from build123d import *

# Parameters (mm, degrees)
SKETCH1_R           = 38.1
BOSS_EXTRUDE1_DEPTH = 12.7
SKETCH2_R           = 24.13
CUT_EXTRUDE1_DEPTH  = 5.08


with BuildPart() as part:
    # Sketch1 → Boss-Extrude1 (new body)
    with BuildSketch(Plane(origin=(0, 0, 0), x_dir=(1, 0, 0), z_dir=(0, 1, 0))):
        with Locations(Location((0, 0, 0), (0, 0, 270))):
            Circle(SKETCH1_R)
    boss_extrude1 = extrude(amount=BOSS_EXTRUDE1_DEPTH)

    # Sketch2 → Cut-Extrude1 (cut)
    with BuildSketch(Plane(origin=(0, 12.7, 0), x_dir=(1, 0, 0), z_dir=(0, 1, 0))):
        with Locations(Location((0, 0, 0), (0, 0, 270))):
            Circle(SKETCH2_R)
    cut_extrude1 = extrude(amount=-CUT_EXTRUDE1_DEPTH, mode=Mode.SUBTRACT)

    # Mirror1: Boss-Extrude1, Cut-Extrude1 across plane
    add(boss_extrude1.mirror(Plane.ZX))
    add(cut_extrude1.mirror(Plane.ZX), mode=Mode.SUBTRACT)


solid = part.part
For this review, take the finished solid that the model builds, in its own axes (mm). A direction names the side the tool comes from. Round coordinates to 2 decimals unless told otherwise and drop trailing zeros. Order: outer loops, then holes, each group sorted by start corner. A loop starts at its lowest first (then second) coordinate and runs counter-clockwise, first axis right, second up. Notation, with made-up numbers: (14.5, 84.25) -> (67.5, 84.25) arc R24 cw to (67.5, 106.25) -> close; hole circle Ø4 at (-17, 50). An arc over 180 degrees is marked (long way). Write item = value, one per line. Start each with the question number.
1) Take a section at D-D on y = -5.75. State the section outline as (x, z) points.
2) The part is to be moulded in two halves that separate along X. For faces 1 (the face through (-25, -12.7, -1)), 2 (the face through (0, 7.62, 0)), 3 (the face through (-23.183, 0.178, -30.235)), 4 (the face through (7.248, 10.196, 23.016)), say which applies: +X half, -X half, draft (parallel to the pull), parting line (faces both ways), or undercut.
3) To check wall thickness, follow line 1 (X direction, y = -8.7, z = 0); line 2 (Y direction, x = -13, z = 0.5); line 3 (Z direction, x = -4.5, y = 8). State the ranges of each line that lie inside material, in increasing order. Write a range as from..to.
4) Insertion check: pin 1 (10 mm diameter, centred on y = 1, z = -17, fed in from -X); pin 2 (1.5 mm diameter, centred on y = 6.5, z = -1.5, fed in from -X); pin 3 (4 mm diameter, centred on x = 18, z = -14.5, fed in from -Y); pin 4 (2 mm diameter, centred on x = 3, z = -4, fed in from -Y). Each pin has a flat end and moves straight along its axis. Give the tip position at first contact, or say it passes through.
5) Tool access review of faces 5 (the face through (-25, 12.7, -1)), 6 (the face through (7.248, -10.196, 23.016)): name each direction out of +Z, -Z, +X, -X, +Y, -Y from which nothing blocks a thin tool from reaching the whole face with its end or side.
6) Take a section at A-A on x = 0. State the section outline as (y, z) points.
7) Take a section at B-B on z = 0. State the section outline as (x, y) points.
8) Take a section at C-C on y = 10. State the section outline as (x, z) points.
Verdict:
q1.outline = circle Ø76.2 at (0, 0)
q2.face_1 = draft
q2.face_2 = undercut
q2.face_3 = parting line
q2.face_4 = undercut
q3.line_1 = -38.1..-24.13, 24.13..38.1
q3.line_2 = -7.62..7.62
q3.line_3 = -37.83..-23.71, 23.71..37.83
q4.pin_1 = -36.16
q4.pin_2 = -38.09
q4.pin_3 = -12.7
q4.pin_4 = -7.62
q5.face_5 = +Z, -Z, +X, -X, +Y
q5.face_6 = -Y
q6.outline = (-12.7, -38.1) -> (12.7, -38.1) -> (12.7, -24.13) -> (7.62, -24.13) -> (7.62, 24.13) -> (12.7, 24.13) -> (12.7, 38.1) -> (-12.7, 38.1) -> (-12.7, 24.13) -> (-7.62, 24.13) -> (-7.62, -24.13) -> (-12.7, -24.13) -> close
q7.outline = (-38.1, -12.7) -> (-24.13, -12.7) -> (-24.13, -7.62) -> (24.13, -7.62) -> (24.13, -12.7) -> (38.1, -12.7) -> (38.1, 12.7) -> (24.13, 12.7) -> (24.13, 7.62) -> (-24.13, 7.62) -> (-24.13, 12.7) -> (-38.1, 12.7) -> close
q8.outline = circle Ø76.2 at (0, 0); hole circle Ø48.26 at (0, 0)
